from build123d import *

# Parameters (mm, degrees)
SKETCH1_W                      = 100
SKETCH1_H                      = 60
BOSS_EXTRUDE1_DEPTH            = 10
CBORE_FOR_M3_SHCS1_D           = 3.6
CBORE_FOR_M3_SHCS1_CBORE_D     = 6.5
CBORE_FOR_M3_SHCS1_CBORE_DEPTH = 3
CUT_EXTRUDE1_REACH             = 61.161
SKETCH5_R                      = 3
SKETCH5_R_2                    = 1.5
FILLET1_R                      = 6


with BuildPart() as part:
    # Sketch1 → Boss-Extrude1 (new body)
    with BuildSketch(Plane(origin=(0, 0, 0), x_dir=(1, 0, 0), z_dir=(0, 1, 0))):
        Rectangle(SKETCH1_W, SKETCH1_H)
    extrude(amount=BOSS_EXTRUDE1_DEPTH)

    # CBORE for M3 SHCS1 (through all)
    with Locations(Plane(origin=(0, 0, 0), x_dir=(-1, 0, 0), z_dir=(0, -1, 0))):
        with Locations((-18, -15), (18, -15)):
            CounterBoreHole(CBORE_FOR_M3_SHCS1_D / 2, CBORE_FOR_M3_SHCS1_CBORE_D / 2, CBORE_FOR_M3_SHCS1_CBORE_DEPTH)

    # Sketch5 → Cut-Extrude1 (cut, up to next)
    with BuildSketch(Plane(origin=(0, 0, 0), x_dir=(-1, 0, 0), z_dir=(0, -1, 0)), mode=Mode.PRIVATE) as cut_extrude1_sk1:
        with Locations(Location((0, 15, 0), (0, 0, 90))):
            Circle(SKETCH5_R)
    cut_extrude1_tool1 = extrude(cut_extrude1_sk1.sketch, amount=-CUT_EXTRUDE1_REACH, mode=Mode.PRIVATE) & part.part
    # Sketch5 → Cut-Extrude1 (cut, up to next)
    with BuildSketch(Plane(origin=(0, 0, 0), x_dir=(-1, 0, 0), z_dir=(0, -1, 0)), mode=Mode.PRIVATE) as cut_extrude1_sk2:
        with Locations(Location((32.5, 15, 0), (0, 0, 90))):
            Circle(SKETCH5_R_2)
    cut_extrude1_tool2 = extrude(cut_extrude1_sk2.sketch, amount=-CUT_EXTRUDE1_REACH, mode=Mode.PRIVATE) & part.part
    # Sketch5 → Cut-Extrude1 (cut, up to next)
    with BuildSketch(Plane(origin=(0, 0, 0), x_dir=(-1, 0, 0), z_dir=(0, -1, 0)), mode=Mode.PRIVATE) as cut_extrude1_sk3:
        with Locations(Location((-32.5, 15, 0), (0, 0, 90))):
            Circle(SKETCH5_R_2)
    cut_extrude1_tool3 = extrude(cut_extrude1_sk3.sketch, amount=-CUT_EXTRUDE1_REACH, mode=Mode.PRIVATE) & part.part
    add(cut_extrude1_tool1.solids().sort_by_distance((0, 0, -15))[0], mode=Mode.SUBTRACT)
    add(cut_extrude1_tool2.solids().sort_by_distance((-32.5, 0, -15))[0], mode=Mode.SUBTRACT)
    add(cut_extrude1_tool3.solids().sort_by_distance((32.5, 0, -15))[0], mode=Mode.SUBTRACT)

    # Fillet1
    fillet1_edges = [part.edges().sort_by_distance(p)[0] for p in [
        (50, 5, 30),
        (-50, 5, 30),
        (-50, 5, -30),
        (50, 5, -30),
    ]]
    fillet(fillet1_edges, radius=FILLET1_R)


solid = part.part
Read the model definition and answer for the solid it produces. Units are mm, in the model's axes. A direction names the side the tool comes from. Round coordinates to 2 decimals unless told otherwise and drop trailing zeros. Write each loop counter-clockwise with the first axis right and the second up, starting at its lowest first coordinate (ties: lowest second). Pieces come first, ordered by that corner, then holes.
1. The part is cut by section B-B, the plane z = 15. Determine the outline of the cut face in (x, y), then the cut area to 3 significant figures.
2. The part is cut by section C-C, the plane y = 4. Determine the outline of the cut face in (x, z), then the cut area to 3 significant figures.
3. Straight lines are drawn through the part: L1, parallel to X at y = 1.35, z = 15; L2, parallel to X at y = 2.75, z = -15; L3, parallel to X at y = 0.5, z = 16. For each, find the intervals that lie inside material, in ascending order.
4. The part is cut by section A-A, the plane x = -18. Determine the outline of the cut face in (y, z).
5. Which of the six approach directions +Z, -Z, +X, -X, +Y, -Y give full straight-line access (tool end or side, diameter ignored) to faces 1 (the face through (-48.289, 5.07, 28.196)), 2 (the face through (16.6, 3, 16.4))?
6. The part is cut by section D-D, the plane x = 32.5. Determine the outline of the cut face in (y, z).
7. Determine the mould class of faces 3 (the face through (-1, 10, 0)), 4 (the face through (50, 5, 0)), 5 (the face through (31.6, 4.9, -13.8)) for opening direction X: pulls with the +X half, pulls with the -X half, needs draft (parallel to the pull), parting line crosses it, or undercut.
8. Given pin 1 Ø10.5 at (x, z) = (18, 15) entering from +Y; pin 2 Ø2.5 at (x, z) = (32.5, -15) entering from +Y; pin 3 Ø4.5 at (x, z) = (-18, 15) entering from -Y, each flat-ended and moving along its own axis, determine where each tip first touches the part or whether it passes through.
Values:
1. outline: (-50, 0) - (-21.25, 0) - (-21.25, 3) - (-19.8, 3) - (-19.8, 10) - (-50, 10) - close; (-16.2, 3) - (-14.75, 3) - (-14.75, 0) - (14.75, 0) - (14.75, 3) - (16.2, 3) - (16.2, 10) - (-16.2, 10) - close; (19.8, 3) - (21.25, 3) - (21.25, 0) - (50, 0) - (50, 10) - (19.8, 10) - close
1. area: 911 mm2
2. outline: (-50, -24) arc R6 ccw to (-44, -30) - (44, -30) arc R6 ccw to (50, -24) - (50, 24) arc R6 ccw to (44, 30) - (-44, 30) arc R6 ccw to (-50, 24) - close; hole circle Ø3 at (-32.5, -15); hole circle Ø3.6 at (-18, 15); hole circle Ø6 at (0, -15); hole circle Ø3.6 at (18, 15); hole circle Ø3 at (32.5, -15)
2. area: 5,910 mm2
3. L1: x = -50 to -21.25, -14.75 to 14.75, 21.25 to 50
3. L2: x = -50 to -34, -31 to -3, 3 to 31, 34 to 50
3. L3: x = -50 to -21.09, -14.91 to 14.91, 21.09 to 50
4. outline: (0, -30) - (10, -30) - (10, 13.2) - (3, 13.2) - (3, 11.75) - (0, 11.75) - close; (0, 18.25) - (3, 18.25) - (3, 16.8) - (10, 16.8) - (10, 30) - (0, 30) - close
5. face 1: +Z, -X, +Y, -Y
5. face 2: -Y
6. outline: (0, -30) - (10, -30) - (10, -16.5) - (0, -16.5) - close; (0, -13.5) - (10, -13.5) - (10, 30) - (0, 30) - close
7. face 3: needs draft
7. face 4: pulls with the +X half
7. face 5: undercut
8. pin 1: stops at y = 10
8. pin 2: passes through
8. pin 3: stops at y = 3
